```python
from build123d import *

# Parameters (mm, degrees)
F0_W     = 140
F0_H     = 100
F1_DEPTH = 10
F2_SIZE2 = 19.99999
F2_SIZE  = 19.99999
F3_SIZE2 = 19.99999
F3_SIZE  = 19.99999


# Not quite as in the source:
# - a fillet or chamfer is up to 0.001 mm smaller than in the source, because OpenCascade refuses the exact size


with BuildPart() as f1:
    # F0 (on Front) → F1 (new body, symmetric)
    with BuildSketch(Plane.XZ):
        with Locations((70, 50)):
            Rectangle(F0_W, F0_H)
    extrude(amount=F1_DEPTH, both=True)

    # F2 (size 20 and 20 in the source; OpenCascade refuses exactly that, so slightly less here)
    f2_edges = [f1.edges().sort_by_distance(p)[0] for p in [
        (140, -10, 50),
    ]]
    chamfer(f2_edges, length=F2_SIZE, length2=F2_SIZE2)

    # F3 (size 20 and 20 in the source; OpenCascade refuses exactly that, so slightly less here)
    f3_edges = [f1.edges().sort_by_distance(p)[0] for p in [
        (0, -10, 50),
    ]]
    chamfer(f3_edges, length=F3_SIZE, length2=F3_SIZE2)


solid = f1.part
```
Verification items for the finished model (mm, model axes). Coordinates: 2 decimals unless noted, no trailing zeros. Loops run counter-clockwise (first coordinate to the right, second up) from the corner with the lowest first, then second, coordinate; pieces in that order, holes last. Notation, with made-up numbers: (51.25, 10) - (94.25, 10) arc R26 cw to (94.25, 32) - close; hole circle Ø8 at (-13, 64.25). An arc over 180 degrees is marked (long way). Put each result on its own line as item: value.
Item 1: Gauge pin test, flat ends, axial feed: pin 1 Ø10 at (y, z) = (-2, 41.5) entering from +X; pin 2 Ø3 at (x, y) = (89, 6.5) entering from -Z; pin 3 Ø3 at (y, z) = (7.5, 58.5) entering from -X; pin 4 Ø5 at (y, z) = (1, 52.5) entering from +X. Record the tip position at first contact, or that the pin passes through.
Conclusion:
pin 1: stops at x = 133
pin 2: stops at z = 0
pin 3: stops at x = 1
pin 4: stops at x = 133.5
Item 2: Scan lines: line 1 along X through (y, z) = (-8.75, 36); line 2 along X through (y, z) = (4.75, 95.5); line 3 along Y through (x, z) = (121, 17). Record each from-to range of solid material in increasing order.
Conclusion:
line 1: x = 18.75 to 121.25
line 2: x = 5.25 to 134.75
line 3: y = -9 to 10
Item 3: Section check C-C (x = 126). Enter the section's corners in (y, z).
Conclusion:
outline: (-4, 0) - (10, 0) - (10, 100) - (-4, 100) - close
Item 4: Section check A-A (y = -5.5). Enter the section's corners in (x, z).
Conclusion:
outline: (15.5, 0) - (124.5, 0) - (124.5, 100) - (15.5, 100) - close
